Check sheet for the modelled part. Datum: model origin and axes. Units: mm. Round coordinates to 2 decimals unless told otherwise and drop trailing zeros. Order: outer loops, then holes, each group sorted by start corner. A loop starts at its lowest first (then second) coordinate and runs counter-clockwise, first axis right, second up.
Q1. Cross-section at A-A on y = -15.8. Record the cut outline in (x, z), then the cut area to 3 significant figures.
Q2. Depth check by flat-ended pin: P1, Ø4, axis at x = 49, y = -15.8, coming from the +Z side; P2, Ø3, axis at x = -48, y = -15.8, coming from the +Z side. Enter the tip coordinate at first touch or a pass-through.
Q3. Scan lines: probe 1 along Y at (x, z) = (3, 0.4); probe 2 along Y at (x, z) = (-48, 0.75); probe 3 along X at (y, z) = (9, 0.55). Record each from-to range of solid material in increasing order.
Q4. Cross-section at B-B on x = -48. Record the cut outline in (y, z).
Q5. Cross-section at C-C on y = -9.5. Record the cut outline in (x, z), then the cut area to 3 significant figures.
Q6. Mould release check, pull along X, two halves, no side actions. Record for faces 1 (the cylindrical face through (47.522, 14.216, 0.493)), 2 (the cylindrical face through (-54.43, 18.2, 0.51)), 3 (the cylindrical face through (54.4, -18.23, 0.51)): +X half, -X half, draft (parallel to the pull), parting line (faces both ways), or undercut.
Q7. Cross-section at D-D on z = 0.2. Record the cut outline in (x, y), then the cut area to 3 significant figures.
from build123d import *

# Parameters (mm, degrees)
SKETCH_1_W          = 110
SKETCH_1_H          = 37.6
EXTRUDE_1_DEPTH     = 1
SKETCH_2_R          = 1.55
CUT_EXTRUDE_1_DEPTH = 10
FILLET_1_R          = 2
SKETCH_3_W          = 57.499999899
SKETCH_3_H          = 18
CUT_EXTRUDE_2_DEPTH = 10
SKETCH_4_W          = 2
SKETCH_4_H          = 18
EXTRUDE_2_DEPTH     = 1
FILLET_2_R          = 1.5
SKETCH_5_W          = 88
SKETCH_5_H          = 25.6
CUT_EXTRUDE_3_DEPTH = 10
SKETCH_6_W          = 88
SKETCH_6_H          = 5
EXTRUDE_3_DEPTH     = 1
FILLET_3_R          = 1.1


with BuildPart() as part:
    # 草图1 → 凸台-拉伸1 (new body)
    with BuildSketch(Plane.XY):
        Rectangle(SKETCH_1_W, SKETCH_1_H)
    extrude(amount=EXTRUDE_1_DEPTH)

    # 草图2 → 切除-拉伸1 (cut)
    with BuildSketch(Plane(origin=(0, 0, 0), x_dir=(-1, 0, 0), z_dir=(0, 0, -1))):
        with Locations((48, 13.75)):
            Circle(SKETCH_2_R)
        with Locations((48, -15.8)):
            Circle(SKETCH_2_R)
        with Locations((-49, -15.8)):
            Circle(SKETCH_2_R)
        with Locations((-49, 13.75)):
            Circle(SKETCH_2_R)
    extrude(amount=-CUT_EXTRUDE_1_DEPTH, mode=Mode.SUBTRACT)

    # 圆角1
    fillet_1_edges = [part.edges().sort_by_distance(p)[0] for p in [
        (55, -18.8, 0.5),
        (-55, -18.8, 0.5),
        (-55, 18.8, 0.5),
        (55, 18.8, 0.5),
    ]]
    fillet(fillet_1_edges, radius=FILLET_1_R)

    # 草图3 → 切除-拉伸2 (cut)
    with BuildSketch(Plane(origin=(0, 0, 0), x_dir=(-1, 0, 0), z_dir=(0, 0, -1))):
        with Locations((9.655484107, -3.8)):
            Rectangle(SKETCH_3_W, SKETCH_3_H)
    extrude(amount=-CUT_EXTRUDE_2_DEPTH, mode=Mode.SUBTRACT)

    # 草图4 → 凸台-拉伸2 (add)
    with BuildSketch(Plane(origin=(0, 0, 0), x_dir=(-1, 0, 0), z_dir=(0, 0, -1))):
        with Locations((-10.094515843, -3.8)):
            Rectangle(SKETCH_4_W, SKETCH_4_H)
        with Locations((-0.094515843, -3.8)):
            Rectangle(SKETCH_4_W, SKETCH_4_H)
        with Locations((9.905484157, -3.8)):
            Rectangle(SKETCH_4_W, SKETCH_4_H)
        with Locations((19.905484157, -3.8)):
            Rectangle(SKETCH_4_W, SKETCH_4_H)
        with Locations((29.905484157, -3.8)):
            Rectangle(SKETCH_4_W, SKETCH_4_H)
    extrude(amount=-EXTRUDE_2_DEPTH)

    # 圆角2
    fillet_2_edges = [part.edges().sort_by_distance(p)[0] for p in [
        (-8.905484157, -12.8, 0.5),
        (-8.905484157, 5.2, 0.5),
        (-10.905484157, 5.2, 0.5),
        (-10.905484157, -12.8, 0.5),
        (-18.905484157, -12.8, 0.5),
        (-18.905484157, 5.2, 0.5),
        (-20.905484157, 5.2, 0.5),
        (-20.905484157, -12.8, 0.5),
        (-28.905484157, -12.8, 0.5),
        (-28.905484157, 5.2, 0.5),
        (-30.905484157, 5.2, 0.5),
        (-30.905484157, -12.8, 0.5),
        (-38.405484056, 5.2, 0.5),
        (-38.405484056, -12.8, 0.5),
        (19.094515843, -12.8, 0.5),
        (19.094515843, 5.2, 0.5),
        (11.094515843, 5.2, 0.5),
        (9.094515843, 5.2, 0.5),
        (9.094515843, -12.8, 0.5),
        (11.094515843, -12.8, 0.5),
        (1.094515843, -12.8, 0.5),
        (1.094515843, 5.2, 0.5),
        (-0.905484157, 5.2, 0.5),
        (-0.905484157, -12.8, 0.5),
    ]]
    fillet(fillet_2_edges, radius=FILLET_2_R)

    # 草图5 → 切除-拉伸3 (cut)
    with BuildSketch(Plane.XY.offset(1)):
        Rectangle(SKETCH_5_W, SKETCH_5_H)
    extrude(amount=-CUT_EXTRUDE_3_DEPTH, mode=Mode.SUBTRACT)

    # 草图6 → 凸台-拉伸3 (add)
    with BuildSketch(Plane.XY.offset(1)):
        Rectangle(SKETCH_6_W, SKETCH_6_H)
    extrude(amount=-EXTRUDE_3_DEPTH)

    # 圆角3
    fillet_3_edges = [part.edges().sort_by_distance(p)[0] for p in [
        (44, -12.8, 0.5),
        (44, 12.8, 0.5),
        (-44, -12.8, 0.5),
        (-44, 12.8, 0.5),
        (-44, 2.5, 0.5),
        (-44, -2.5, 0.5),
        (44, -2.5, 0.5),
        (44, 2.5, 0.5),
    ]]
    fillet(fillet_3_edges, radius=FILLET_3_R)


solid = part.part
Results found:
1. outline: (-55, 0) - (-49.55, 0) - (-49.55, 1) - (-55, 1) - close; (-46.45, 0) - (47.45, 0) - (47.45, 1) - (-46.45, 1) - close; (50.55, 0) - (55, 0) - (55, 1) - (50.55, 1) - close
1. area: 104 mm2
2. P1: stops at z = 1
2. P2: passes through
3. probe 1: y = -18.8 to -12.8, -2.5 to 2.5, 12.8 to 18.8
3. probe 2: y = -18.8 to -17.35, -14.25 to 12.2, 15.3 to 18.8
3. probe 3: x = -55 to -44, 44 to 55
4. outline: (-18.8, 0) - (-17.35, 0) - (-17.35, 1) - (-18.8, 1) - close; (-14.25, 0) - (12.2, 0) - (12.2, 1) - (-14.25, 1) - close; (15.3, 0) - (18.8, 0) - (18.8, 1) - (15.3, 1) - close
5. outline: (-55, 0) - (-44, 0) - (-44, 1) - (-55, 1) - close; (44, 0) - (55, 0) - (55, 1) - (44, 1) - close
5. area: 22.0 mm2
6. face 1: undercut
6. face 2: -X half
6. face 3: +X half
7. outline: (-55, -16.8) arc R2 ccw to (-53, -18.8) - (53, -18.8) arc R2 ccw to (55, -16.8) - (55, 16.8) arc R2 ccw to (53, 18.8) - (-53, 18.8) arc R2 ccw to (-55, 16.8) - close; hole circle Ø3.1 at (-48, -15.8); hole circle Ø3.1 at (-48, 13.75); hole (-44, -11.7) arc R1.1 ccw to (-42.9, -12.8) - (42.9, -12.8) arc R1.1 ccw to (44, -11.7) - (44, -3.6) arc R1.1 ccw to (42.9, -2.5) - (-42.9, -2.5) arc R1.1 ccw to (-44, -3.6) - close; hole (-44, 3.6) arc R1.1 ccw to (-42.9, 2.5) - (42.9, 2.5) arc R1.1 ccw to (44, 3.6) - (44, 11.7) arc R1.1 ccw to (42.9, 12.8) - (-42.9, 12.8) arc R1.1 ccw to (-44, 11.7) - close; hole circle Ø3.1 at (49, -15.8); hole circle Ø3.1 at (49, 13.75)
7. area: 2,290 mm2
